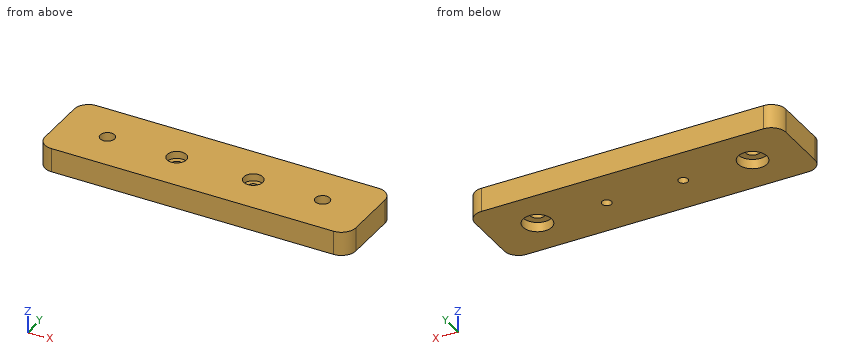
from build123d import *

# Parameters (mm, degrees)
SKETCH1_W           = 65
SKETCH1_H           = 17
SKETCH1_R           = 1.5
SKETCH1_R_2         = 1
BOSS_EXTRUDE1_DEPTH = 5
FILLET1_R           = 3
SKETCH3_R           = 2
CUT_EXTRUDE2_DEPTH  = 1.5
SKETCH4_R           = 3
CUT_EXTRUDE3_DEPTH  = 2


with BuildPart() as part:
    # Sketch1 → Boss-Extrude1 (new body)
    with BuildSketch(Plane.XY):
        with Locations((32.5, 8.5)):
            Rectangle(SKETCH1_W, SKETCH1_H)
        with Locations((55, 8.5)):
            Circle(SKETCH1_R, mode=Mode.SUBTRACT)
        with Locations((10, 8.5)):
            Circle(SKETCH1_R, mode=Mode.SUBTRACT)
        with Locations((24.5, 8.5)):
            Circle(SKETCH1_R_2, mode=Mode.SUBTRACT)
        with Locations((40.5, 8.5)):
            Circle(SKETCH1_R_2, mode=Mode.SUBTRACT)
    extrude(amount=BOSS_EXTRUDE1_DEPTH)

    # Fillet1
    fillet1_edges = [part.edges().sort_by_distance(p)[0] for p in [
        (0, 17, 2.5),
        (65, 17, 2.5),
        (65, 0, 2.5),
        (0, 0, 2.5),
    ]]
    fillet(fillet1_edges, radius=FILLET1_R)

    # Sketch3 → Cut-Extrude2 (cut)
    with BuildSketch(Plane.XY.offset(5)):
        with Locations((24.5, 8.5)):
            Circle(SKETCH3_R)
        with Locations((40.5, 8.5)):
            Circle(SKETCH3_R)
    extrude(amount=-CUT_EXTRUDE2_DEPTH, mode=Mode.SUBTRACT)

    # Sketch4 → Cut-Extrude3 (cut)
    with BuildSketch(Plane(origin=(0, 0, 0), x_dir=(-1, 0, 0), z_dir=(0, 0, -1))):
        with Locations((-55, 8.5)):
            Circle(SKETCH4_R)
        with Locations((-10, 8.5)):
            Circle(SKETCH4_R)
    extrude(amount=-CUT_EXTRUDE3_DEPTH, mode=Mode.SUBTRACT)


solid = part.part
Geometry: final body of the model. Coordinates: model frame, mm. Round coordinates to 2 decimals unless told otherwise and drop trailing zeros. Loops run counter-clockwise (first coordinate to the right, second up) from the corner with the lowest first, then second, coordinate; pieces in that order, holes last. Notation, with made-up numbers: (-21, -26.75) - (-17, -26.75) arc R11 cw to (-17, -21.75) - close; hole circle Ø4 at (30, -33.5). An arc over 180 degrees is marked (long way). Write each question's results on one line, items separated by ' | '. Start each with the question number.
1) Cut plane A-A on x = 40.5. Return loops of the section in (y, z).
2) First-contact query: P1, Ø1.2, axis at x = 24, y = 8.5, coming from the +Z side; P2, Ø3.5, axis at x = 10, y = 8.5, coming from the -Z side. Flat tips, straight axial feed; report the tip coordinate or a pass-through.
3) Cut plane C-C on x = 10. Return loops of the section in (y, z).
4) Line query: probe 1 along X at (y, z) = (8.5, 2.75); probe 2 along Y at (x, z) = (55, 0.6); probe 3 along X at (y, z) = (14.25, 0.75). Output: solid intervals per line, ascending. Write a range as [from, to].
5) Cut plane B-B on y = 8.5. Count the separate pieces of the cut face and the enclosed holes in it, then the cut area to 3 significant figures.
Verdict:
1) outline: (0, 0) - (7.5, 0) - (7.5, 3.5) - (6.5, 3.5) - (6.5, 5) - (0, 5) - close; (9.5, 0) - (17, 0) - (17, 5) - (10.5, 5) - (10.5, 3.5) - (9.5, 3.5) - close
2) P1: stops at z = 3.5 | P2: stops at z = 2
3) outline: (0, 0) - (5.5, 0) - (5.5, 2) - (7, 2) - (7, 5) - (0, 5) - close; (10, 2) - (11.5, 2) - (11.5, 0) - (17, 0) - (17, 5) - (10, 5) - close
4) probe 1: x = [0, 8.5], [11.5, 23.5], [25.5, 39.5], [41.5, 53.5], [56.5, 65] | probe 2: y = [0, 5.5], [11.5, 17] | probe 3: x = [0.01, 64.99]
5) separate pieces: 5 | enclosed holes: 0 | area: 257 mm2
